The listing builds one solid part. Answer for the finished solid, in the listing's coordinates (mm). Face numbers are marked on the shaded views. A direction names the side the tool comes from. Round coordinates to 2 decimals unless told otherwise and drop trailing zeros. Order: outer loops, then holes, each group sorted by start corner. A loop starts at its lowest first (then second) coordinate and runs counter-clockwise, first axis right, second up. Notation, with made-up numbers: (-20, 36.25) - (-16, 36.25) arc R17 cw to (-16, 44.25) - close; hole circle Ø8 at (84, -12.75). An arc over 180 degrees is marked (long way). Write item = value, one per line.
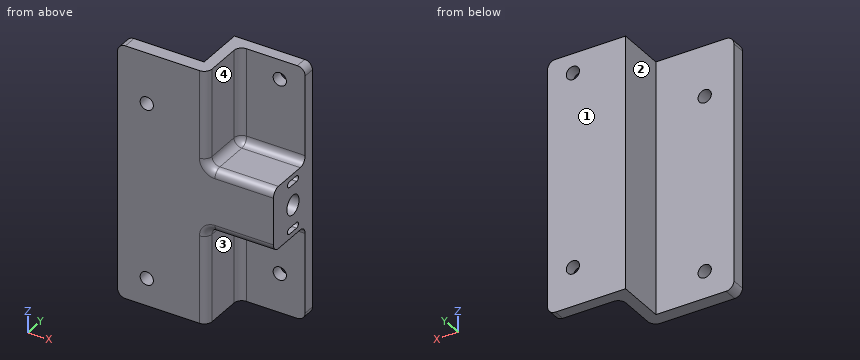
Autodesk Inventor part; units mm, degrees
ref_plane "YZ Plane" through (0, 0, 0) normal (1, 0, 0) x (0, 1, 0)
ref_plane "XZ Plane" through (0, 0, 0) normal (0, 1, 0) x (-1, 0, 0)
ref_plane "XY Plane" through (0, 0, 0) normal (0, 0, 1) x (1, 0, 0)
sketch "Sketch1" plane through (0, 0, 0) normal (0, 1, 0) x (-1, 0, 0)
  line L0 (0, 0) -> (40, 0)
  line L1 (40, 0) -> (40, -65)
  line L2 (40, -65) -> (0, -65)
  line L3 (0, -65) -> (0, 0)
  dimension "d0" = 40
  dimension "d1" = 65
extrude "Extrusion1" add sketch "Sketch1" along normal blind 16
sketch "Sketch2" plane through (-40, 0, 0) normal (0, 0, 1) x (1, 0, 0)
  line L0 (0, 16) -> (40, 16)
  line L1 (0, 16) -> (20, 16)
  line L2 (20, 16) -> (20, 3.5)
  line L3 (20, 3.5) -> (0, 3.5)
  line L4 (0, 3.5) -> (0, 16)
  line L5 (40, 0) -> (0, 0)
  dimension "d4" = 20
  dimension "d5" = 3.5
extrude "Extrusion2" cut sketch "Sketch2" against normal through all
sketch "Sketch3" plane through (0, 0, 0) normal (0, -1, 0) x (1, 0, 0)
  line L0 (-32.5, -58) -> (-32.5, -13) construction
  line L1 (-6.5, -55) -> (-6.5, -5) construction
  line L2 (-40, -65) -> (0, -65) construction
  line L3 (0, 0) -> (-40, 0) construction
  line L4 (0, -65) -> (0, 0) construction
  line L5 (-40, 0) -> (-40, -65) construction
  dimension "d8" = 45
  dimension "d9" = 50
  dimension "d10" = 7
  dimension "d11" = 5
  dimension "d12" = 6.5
  dimension "d13" = 7.5
hole "Hole1" at (-32.5, 0, -58) at (-32.5, 0, -13) at (-6.5, 0, -55) at (-6.5, 0, -5) direction (0, 1, 0) diameter 3.4 end through all
sketch "Sketch4" plane through (0, 0, 0) normal (1, 0, 0) x (0, 0, -1)
  line L0 (38.5, 6.5) -> (38.5, 9.5) construction
  line L1 (39.25, 6.5) -> (39.25, 9.5)
  line L2 (37.75, 9.5) -> (37.75, 6.5)
  arc A0 (37.75, 6.5) -> (39.25, 6.5) centre (38.5, 6.5) ccw
  arc A1 (39.25, 9.5) -> (37.75, 9.5) centre (38.5, 9.5) ccw
  line L3 (26.5, 6.5) -> (26.5, 9.5) construction
  line L4 (27.25, 6.5) -> (27.25, 9.5)
  line L5 (25.75, 9.5) -> (25.75, 6.5)
  arc A2 (25.75, 6.5) -> (27.25, 6.5) centre (26.5, 6.5) ccw
  arc A3 (27.25, 9.5) -> (25.75, 9.5) centre (26.5, 9.5) ccw
  line L6 (0, 0) -> (0, 16) construction
  line L7 (65, 0) -> (65, 16) construction
  line L8 (38.5, 8) -> (26.5, 8) construction
  line L9 (65, 0) -> (0, 0) construction
  line L10 (0, 16) -> (65, 16) construction
  line L11 (65, 0) -> (40.5, 0)
  line L12 (40.5, 0) -> (40.5, 13)
  line L13 (40.5, 13) -> (65, 13)
  line L14 (65, 13) -> (65, 0)
  line L15 (24.5, 0) -> (0, 0)
  line L16 (0, 0) -> (0, 13)
  line L17 (0, 13) -> (24.5, 13)
  line L18 (24.5, 13) -> (24.5, 0)
  point P0 (32.5, 8)
  dimension "d21" = 12
  dimension "d22" = 6
  dimension "d23" = 65
  dimension "d24" = 32.5
  dimension "d25" = 3
  dimension "d26" = 3
  dimension "d27" = 0.75
  dimension "d28" = 0.75
  dimension "d29" = 0
  dimension "d30" = 16
  dimension "d31" = 8
  dimension "d32" = 3
  dimension "d33" = 3
  dimension "d34" = 16
  dimension "d35" = 8
extrude "Extrusion3" cut sketch "Sketch4" against normal blind 2 contours A0 L2 A1 L1 | A2 L5 A3 L4
extrude "Extrusion4" cut sketch "Sketch4" against normal blind 17 contours L11 L12 L13 L14 | L15 L16 L17 L18
fillet "Fillet1" radius 2 14 edges at (-8.5, 0, -40.5) (-8.5, 0, -24.5) (-40, 1.75, -65) (-40, 1.75, 0) (0, 14.5, 0) (0, 14.5, -65) (-17, 0, -52.75) (-17, 0, -12.25) (-17, 6.5, -40.5) (-17, 6.5, -24.5) (-17, 13, -52.75) (-8.5, 13, -40.5) (-17, 13, -12.25) (-8.5, 13, -24.5)
hole "Hole2" at (0, 8, -32.5) direction (-1, 0, 0) diameter 4.978 depth 10 tip angle 118
equation "\"d26\" = d25"
equation "\"d28\" = d27"
properties part number "Dual Camera Mount"
Q1. Section A-A on z = -5 is taken. Determine the outline of the cut face in (x, y), then the cut area to 3 significant figures.
Model answer:
outline = (-40, 0) - (-19, 0) arc R2 ccw to (-17, 2) - (-17, 11) arc R2 cw to (-15, 13) - (-8.2, 13) - (-8.2, 16) - (-20, 16) - (-20, 3.5) - (-40, 3.5) - close; (-4.8, 13) - (0, 13) - (0, 16) - (-4.8, 16) - close
area = 159 mm^2
Q2. For the marked faces 1, 2, 3 and 4, determine the directions among +Z, -Z, +X, -X, +Y, -Y from which every point of the face is accessible in a straight line to the end or side of a thin tool.
Model answer:
face_1 = +Z, -Z, +X, -X, +Y
face_2 = +Z, -Z, -X, +Y
face_3 = -Z, +X, -Y
face_4 = +Z, +X, -Y
Q3. Section C-C on z = -36 is taken. Determine the outline of the cut face in (x, y).
Model answer:
outline = (-40, 0) - (0, 0) - (0, 16) - (-20, 16) - (-20, 3.5) - (-40, 3.5) - close
Q4. Find the intervals of material crossed by line 1 (Z direction, x = -32.5, y = 1); line 2 (X direction, y = 1.85, z = -13); line 3 (X direction, y = 14.2, z = -5), in increasing order. Write a range as from..to.
Model answer:
line_1 = -65..-59.7, -56.3..-14.7, -11.3..0
line_2 = -40..-34.2, -30.8..-17.01
line_3 = -20..-8.2, -4.8..0
Q5. Flat-ended cylindrical pins translate along their axes: P1, Ø12, axis at x = -21.5, z = -17, coming from the -Y side; P2, Ø1, axis at x = -1, y = 7.5, coming from the -Z side; P3, Ø0.8, axis at y = 7.5, z = -38.5, coming from the +X side; P4, Ø2.5, axis at y = 5, z = -7.5, coming from the +X side. Find the tip coordinate at first contact, or state that the pin passes through.
Model answer:
P1 = 0
P2 = -40.5
P3 = -2
P4 = -17
Q6. Section D-D on z = -13 is taken. Determine the outline of the cut face in (x, y), then the cut area to 3 significant figures.
Model answer:
outline = (-40, 0) - (-34.2, 0) - (-34.2, 3.5) - (-40, 3.5) - close; (-30.8, 0) - (-19, 0) arc R2 ccw to (-17, 2) - (-17, 11) arc R2 cw to (-15, 13) - (0, 13) - (0, 16) - (-20, 16) - (-20, 3.5) - (-30.8, 3.5) - close
area = 157 mm^2
Q7. Section B-B on y = 4.75 is taken. Determine the outline of the cut face in (x, z), then the cut area to 3 significant figures.
Model answer:
outline = (-20, -65) - (-17, -65) - (-17, -42.5) arc R2 cw to (-15, -40.5) - (0, -40.5) - (0, -24.5) - (-15, -24.5) arc R2 cw to (-17, -22.5) - (-17, 0) - (-20, 0) - close
area = 469 mm^2
